Autodesk Inventor part; units mm, degrees
ref_plane "YZ Plane" through (0, 0, 0) normal (1, 0, 0) x (0, 1, 0)
ref_plane "XZ Plane" through (0, 0, 0) normal (0, 1, 0) x (-1, 0, 0)
ref_plane "XY Plane" through (0, 0, 0) normal (0, 0, 1) x (1, 0, 0)
sketch "スケッチ1" plane through (0, 0, 0) normal (0, 0, 1) x (1, 0, 0)
  circle A0 centre (0, 0) radius 16
  dimension "d0" = 32
extrude "押し出し1" add sketch "スケッチ1" along normal blind 13.88
sketch "スケッチ2" plane through (0, 0, 13.88) normal (0, 0, 1) x (1, 0, 0)
  circle A0 centre (0, 0) radius 16
  circle A1 centre (0, 0) radius 10
  circle A2 centre (0, 0) radius 4
  dimension "d3" = 6
  dimension "d4" = 6
extrude "押し出し2" cut sketch "スケッチ2" against normal blind 5.5 contours A1
ref_plane "作業平面1" through (0, 0, 6.94) normal (0, 0, 1) x (1, 0, 0)
mirror "ミラー1" about plane through (0, 0, 6.94) normal (0, 0, 1) of "押し出し2"
sketch "スケッチ3" plane through (0, 0, 13.88) normal (0, 0, 1) x (1, 0, 0)
  point P0 (0, 0)
  point P1 (0, 0)
hole "穴1" at (0, 0, 13.88) direction (0, 0, -1) diameter 4.5 depth 13.88
sketch "スケッチ4" plane through (0, 0, 13.88) normal (0, 0, 1) x (1, 0, 0)
  circle A0 centre (0, 0) radius 2.25
  circle A1 centre (0, 0) radius 4
extrude "押し出し3" add sketch "スケッチ4" along normal blind 1.11
mirror "ミラー2" about plane through (0, 0, 6.94) normal (0, 0, 1) of "押し出し3"
properties part number "wheel" material "ゴム"
Verification items for the finished model (mm, model axes). A direction names the side the tool comes from. Give positions to 0.01 mm unless a question says otherwise; leave off trailing zeros. Write each loop counter-clockwise with the first axis right and the second up, starting at its lowest first coordinate (ties: lowest second). Pieces come first, ordered by that corner, then holes. Notation, with made-up numbers: (-36, -38) - (-29, -38) arc R37 ccw to (-29, -1) - close; hole circle Ø4 at (3.25, -8). An arc over 180 degrees is marked (long way). Put each result on its own line as item: value.
Q1. Section check D-D on z = 7.5. Record the cut outline in (x, y).
Result:
outline: circle Ø32 at (0, 0); hole circle Ø4.5 at (0, 0)
Q2. Scan lines: probe 1 along Y at (x, z) = (0, 10.7); probe 2 along Z at (x, y) = (-0.5, -14); probe 3 along Z at (x, y) = (1, -6.5). Record each from-to range of solid material in increasing order. Write a range as from..to.
Result:
probe 1: -16..-10, -4..-2.25, 2.25..4, 10..16
probe 2: 0..13.88
probe 3: 5.5..8.38
Q3. Set-up check for faces 1 (the face through (2, -2, 14.99)), 2 (the face through (-2.17, 9.76, 2.71)), 3 (the face through (-0.2, -10.4, 13.88)): record each of +Z, -Z, +X, -X, +Y, -Y from which the full face is reachable in a straight line by a thin tool's end or side.
Result:
face 1: +Z, +X, -X, +Y, -Y
face 2: -Z
face 3: +Z
Q4. Section check C-C on z = 10. Record the cut outline in (x, y).
Result:
outline: circle Ø32 at (0, 0); circle Ø8 at (0, 0); hole circle Ø20 at (0, 0); hole circle Ø4.5 at (0, 0)
Q5. Depth check by flat-ended pin: P1, Ø2, axis at x = -12, z = 10, coming from the +Y side; P2, Ø8, axis at x = -9.5, y = 6.5, coming from the +Z side; P3, Ø3, axis at x = -7.5, z = 3.5, coming from the +Y side. Enter the tip coordinate at first touch or a pass-through.
Result:
P1: y = 11.62
P2: z = 13.88
P3: y = 14.83
Q6. Section check A-A on y = 0. Record the cut outline in (x, z), and give its area (3 significant figures).
Result:
outline: (-16, 0) - (-10, 0) - (-10, 5.5) - (-4, 5.5) - (-4, -1.11) - (-2.25, -1.11) - (-2.25, 14.99) - (-4, 14.99) - (-4, 8.38) - (-10, 8.38) - (-10, 13.88) - (-16, 13.88) - close; (2.25, -1.11) - (4, -1.11) - (4, 5.5) - (10, 5.5) - (10, 0) - (16, 0) - (16, 13.88) - (10, 13.88) - (10, 8.38) - (4, 8.38) - (4, 14.99) - (2.25, 14.99) - close
area: 257 mm2
Q7. Mould release check, pull along X, two halves, no side actions. Record for faces 4 (the face through (-0.2, -10.4, 0)), 5 (the face through (-3.47, 15.62, 6.84)), 6 (the face through (-0.867, -3.905, 2.241)): released by +X, released by -X, zero draft, split by the parting line, or undercut.
Result:
face 4: zero draft
face 5: split by the parting line
face 6: undercut
